```python
from build123d import *

# Parameters (mm, degrees)
SKETCH1_R           = 37.5
SKETCH1_R_2         = 3
BOSS_EXTRUDE1_DEPTH = 6
FILLET1_R           = 2
SKETCH2_R           = 1
CUT_EXTRUDE1_DEPTH  = 10
CIRPATTERN1_COUNT   = 4
CUT_EXTRUDE2_START  = -2
SKETCH3_R           = 28.5
SKETCH3_R_2         = 13
CUT_EXTRUDE2_DEPTH  = 2


with BuildPart() as part:
    # Sketch1 → Boss-Extrude1 (new body)
    with BuildSketch(Plane(origin=(0, 0, 0), x_dir=(0, 0, -1), z_dir=(1, 0, 0))):
        Circle(SKETCH1_R)
        with BuildLine():
            ThreePointArc((-12.845232579, -2), (-9.192388155, -9.192388155), (-2, -12.845232579))
            Line((-2, -12.845232579), (-2, -28.429737952))
            ThreePointArc((-2, -28.429737952), (-20.152543264, -20.152543264), (-28.429737952, -2))
            Line((-28.429737952, -2), (-12.845232579, -2))
        make_face(mode=Mode.SUBTRACT)
        with BuildLine():
            ThreePointArc((2, -12.845232579), (9.192388155, -9.192388155), (12.845232579, -2))
            Line((12.845232579, -2), (28.429737952, -2))
            ThreePointArc((28.429737952, -2), (20.152543264, -20.152543264), (2, -28.429737952))
            Line((2, -28.429737952), (2, -12.845232579))
        make_face(mode=Mode.SUBTRACT)
        Circle(SKETCH1_R_2, mode=Mode.SUBTRACT)
        with BuildLine():
            ThreePointArc((-2, 12.845232579), (-9.192388155, 9.192388155), (-12.845232579, 2))
            Line((-12.845232579, 2), (-28.429737952, 2))
            ThreePointArc((-28.429737952, 2), (-20.152543264, 20.152543264), (-2, 28.429737952))
            Line((-2, 28.429737952), (-2, 12.845232579))
        make_face(mode=Mode.SUBTRACT)
        with BuildLine():
            ThreePointArc((12.845232579, 2), (9.192388155, 9.192388155), (2, 12.845232579))
            Line((2, 12.845232579), (2, 28.429737952))
            ThreePointArc((2, 28.429737952), (20.152543264, 20.152543264), (28.429737952, 2))
            Line((28.429737952, 2), (12.845232579, 2))
        make_face(mode=Mode.SUBTRACT)
    extrude(amount=BOSS_EXTRUDE1_DEPTH)

    # Fillet1
    fillet1_edges = [part.edges().sort_by_distance(p)[0] for p in [
        (3, 28.429737952, -2),
        (3, 12.845232579, -2),
        (3, 2, -12.845232579),
        (3, 2, -28.429737952),
        (3, 28.429737952, 2),
        (3, 2, 28.429737952),
        (3, 2, 12.845232579),
        (3, 12.845232579, 2),
        (3, -2, 28.429737952),
        (3, -28.429737952, 2),
        (3, -2, 12.845232579),
        (3, -28.429737952, -2),
        (3, -2, -28.429737952),
        (3, -2, -12.845232579),
        (3, -12.845232579, -2),
    ]]
    fillet(fillet1_edges, radius=FILLET1_R)

    # Sketch2 → Cut-Extrude1 (cut)
    with BuildSketch(Plane(origin=(6, 0, 0), x_dir=(0, 0, -1), z_dir=(1, 0, 0))):
        with BuildLine():
            ThreePointArc((4, 8.062257748), (2.054224947, 8.762428879), (0, 9))
            ThreePointArc((0, 9), (-2.054224947, 8.762428879), (-4, 8.062257748))
            ThreePointArc((-4, 8.062257748), (-3.028509279, 8.016287917), (-2.555555556, 7.166451332))
            ThreePointArc((-2.555555556, 7.166451332), (-2.70571897, 6.639405055), (-3.111111111, 6.270644915))
            ThreePointArc((-3.111111111, 6.270644915), (-1.597730514, 6.815222462), (0, 7))
            ThreePointArc((0, 7), (1.597730514, 6.815222462), (3.111111111, 6.270644915))
            ThreePointArc((3.111111111, 6.270644915), (2.659749139, 7.610895776), (4, 8.062257748))
        make_face()
        with Locations((-3.555555556, 7.166451332)):
            Circle(SKETCH2_R)
        with Locations((3.555555556, 7.166451332)):
            Circle(SKETCH2_R)
    cut_extrude1 = extrude(amount=-CUT_EXTRUDE1_DEPTH, mode=Mode.SUBTRACT)

    # CirPattern1: Cut-Extrude1 ×4 about axis
    cirpattern1_axis = Axis((0, 0, 0), (1, 0, 0))
    for i in range(1, CIRPATTERN1_COUNT):
        add(cut_extrude1.rotate(cirpattern1_axis, i * 360 / CIRPATTERN1_COUNT), mode=Mode.SUBTRACT)

    # Sketch3 → Cut-Extrude2 (cut)
    with BuildSketch(Plane(origin=(6, 0, 0), x_dir=(0, 0, -1), z_dir=(1, 0, 0)).offset(CUT_EXTRUDE2_START)):
        with Locations(Location((0, 0, 0), (0, 0, 171.318398303))):
            Circle(SKETCH3_R)
        with Locations(Location((0, 0, 0), (0, 0, 164.533990047))):
            Circle(SKETCH3_R_2, mode=Mode.SUBTRACT)
    extrude(amount=CUT_EXTRUDE2_DEPTH, mode=Mode.SUBTRACT)


solid = part.part
```
Design review of the part built by this model. Coordinates are the model's own, in mm. A direction names the side the tool comes from. Give positions to 0.01 mm unless a question says otherwise; leave off trailing zeros. Write each loop counter-clockwise with the first axis right and the second up, starting at its lowest first coordinate (ties: lowest second). Pieces come first, ordered by that corner, then holes. Notation, with made-up numbers: (18, 77.25) - (34, 77.25) arc R23 cw to (34, 105.25) - close; hole circle Ø3 at (-1.5, 58.5). An arc over 180 degrees is marked (long way). Return JSON: item names as keys, results as strings. Group by question number.
(1) Machinability: for faces 4 (the flat face through (0, -8, -8)), 5 (the cylindrical face through (2.028, -27.729, 2.715)), which of the approach directions +Z, -Z, +X, -X, +Y, -Y give a long, thin tool a straight path to every point of the face, cutting with its end or side? Answer none if there is none.
(2) We need section A-A, the plane y = 15.5. Give the boundary of the cut face in (x, z).
(3) Insertion check: pin 1 (4.5 mm diameter, centred on y = -19.5, z = 2, fed in from +X); pin 2 (1.2 mm diameter, centred on x = 2, y = 22, fed in from -Z); pin 3 (2 mm diameter, centred on x = 1.5, z = -20.5, fed in from -Y). Each pin has a flat end and moves straight along its axis. Give the tip position at first contact, or say it passes through.
(4) We need section C-C, the plane y = 30. Give the boundary of the cut face in (x, z), then the cut area to 3 significant figures.
(5) We need section B-B, the plane x = 2.8. Give the number of separate pieces and of enclosed holes in the cut face, then the cut area to 3 significant figures.
(6) We need section D-D, the plane y = -11.5. Give the boundary of the cut face in (x, z).
(7) Mouldability with a two-part tool opening along Y and no side actions: class faces 1 (the cylindrical face through (3.04, -6.7, 4.44)), 2 (the flat face through (6, -3, -3)), 3 (the cylindrical face through (2.96, 37.18, 4.88)) as +Y half, -Y half, draft (parallel to the pull), parting line (faces both ways), or undercut.
(8) To check wall thickness, follow probe 1 along Y at (x, z) = (3.1, 23.5); probe 2 along Y at (x, z) = (4.2, -11); probe 3 along Z at (x, y) = (3.1, 5). State the ranges of each line that lie inside material, in increasing order.
Reported:
{
 "1": {"face 4": "+Z, -Z, -X, +Y, -Y", "face 5": "+X, -X"},
 "2": {"outline": "(0, -34.15) - (6, -34.15) - (6, -23.92) - (0, -23.92) - close; (0, -2) - (4, -2) - (4, 2) - (0, 2) - close; (0, 23.92) - (6, 23.92) - (6, 34.15) - (0, 34.15) - close"},
 "3": {"pin 1": "stops at x = 4", "pin 2": "stops at z = -30.79", "pin 3": "stops at y = -32.03"},
 "4": {"outline": "(0, -22.5) - (6, -22.5) - (6, 22.5) - (0, 22.5) - close", "area": "270 mm2"},
 "5": {"separate pieces": "1", "enclosed holes": "9", "area": "2,560 mm2"},
 "6": {"outline": "(0, -35.69) - (6, -35.69) - (6, -26.08) - (0, -26.08) - close; (0, -6.06) - (6, -6.06) - (6, 6.06) - (0, 6.06) - close; (0, 26.08) - (6, 26.08) - (6, 35.69) - (0, 35.69) - close"},
 "7": {"face 1": "undercut", "face 2": "draft", "face 3": "parting line"},
 "8": {"probe 1": "y = -29.22 to -16.12, -2 to 2, 16.12 to 29.22", "probe 2": "y = -35.85 to -26.29, -6.93 to 6.93, 26.29 to 35.85", "probe 3": "z = -37.17 to -28.06, -12 to 12, 28.06 to 37.17"}
}
